Check sheet for the modelled part. Datum: model origin and axes. Units: mm. Give positions to 0.01 mm unless a question says otherwise; leave off trailing zeros. Write each loop counter-clockwise with the first axis right and the second up, starting at its lowest first coordinate (ties: lowest second). Pieces come first, ordered by that corner, then holes. Notation, with made-up numbers: M 76.5,64 L 117.5,64 A19 cw 117.5,101 Z; hole C -11.75,33.5 d5. An arc over 180 degrees is marked long. Use CSV: the item, a comma, the result in double quotes. Start each with the question number.
1. Scan lines: line 1 (X direction, y = 8.5, z = 0.75); line 2 (X direction, y = 17, z = 1.1); line 3 (X direction, y = -8.5, z = 0.3). Record each from-to range of solid material in increasing order.
2. Depth check by flat-ended pin: P1, Ø8, axis at x = 16.5, y = 24.5, coming from the +Z side. Enter the tip coordinate at first touch or a pass-through.
3. Cross-section at D-D, the plane x = -13. Enter the section's corners in (y, z), and give its area (3 significant figures).
4. Cross-section at A-A, the plane y = 0. Enter the section's corners in (x, z), and give its area (3 significant figures).
5. Cross-section at C-C, the plane y = -11. Enter the section's corners in (x, z).
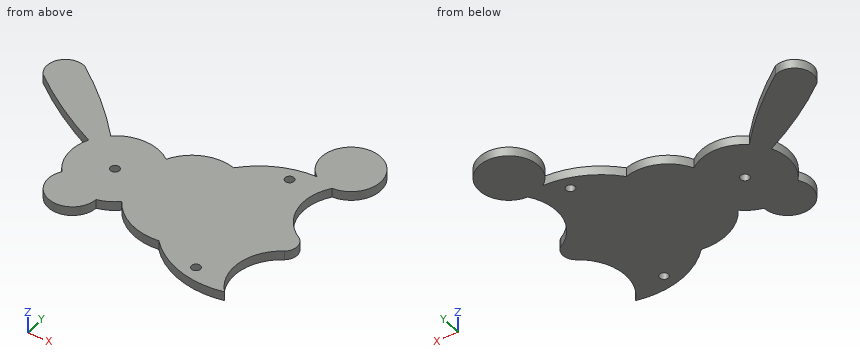
from build123d import *

# Parameters (mm, degrees)
F1_R     = 0.975
F1_R_2   = 5.495
F2_DEPTH = 2


# Not quite as in the source:
# - the program builds the solid bodies; features that only make, move or delete a surface that nothing else refers to are left out


with BuildPart() as f2:
    # F1 (on Top) → F2 (new body)
    with BuildSketch(Plane.XY):
        with BuildLine():
            ThreePointArc((8.3461548541, 12.451567302), (1.7252198574, 12.0948349613), (-3.0867358283, 7.5331334509))
            ThreePointArc((-3.0867358283, 7.5331334509), (-9.1504459177, 9.6196614304), (-15.1782928372, 7.431685066))
            ThreePointArc((-15.1782928372, 7.431685066), (-22.5381757879, 14.8578874844), (-30.6692253798, 21.4307401329))
            ThreePointArc((-30.6692253798, 21.4307401329), (-35.5250947404, 20.1584087851), (-35.4319922626, 15.1394819841))
            ThreePointArc((-35.4319922626, 15.1394819841), (-26.9109452732, 9.1280444677), (-17.7545223506, 4.1374991998))
            ThreePointArc((-17.7545223506, 4.1374991998), (-18.6125164693, -1.2164521529), (-16.4388114376, -6.1839420049))
            ThreePointArc((-16.4388114376, -6.1839420049), (-13.6846503599, -14.1883393203), (-6.7486233515, -9.3357823691))
            ThreePointArc((-6.7486233515, -9.3357823691), (-4.5490625181, -8.4916373097), (-2.6206436977, -7.1381789267))
            ThreePointArc((-2.6206436977, -7.1381789267), (2.5909813664, -11.6392406956), (9.3949967995, -12.7003565431))
            ThreePointArc((9.3949967995, -12.7003565431), (17.7901975829, -17.882711986), (27.6524089277, -18.1528814137))
            ThreePointArc((27.6524089277, -18.1528814137), (24.9662444476, -9.7026669711), (29.7177772104, -2.2163768254))
            ThreePointArc((29.7177772104, -2.2163768254), (30.8881367766, 0.1144698658), (29.7177772104, 2.4453165571))
            ThreePointArc((29.7177772104, 2.4453165571), (24.594325339, 9.3144076758), (26.3560396261, 17.700737901))
            ThreePointArc((26.3560396261, 17.700737901), (27.8220537541, 30.4194435664), (22.2002219007, 18.9168491704))
            ThreePointArc((22.2002219007, 18.9168491704), (14.5953140013, 17.1367848208), (8.3461548541, 12.451567302))
        make_face()
        with BuildLine():
            Line((-17.6755707347, -0.4939858073), (-12.0034380316, -0.4939858073))
            ThreePointArc((-12.0034380316, -0.4939858073), (-10.5336675739, -2.589890275), (-7.9799964747, -2.7682288675))
            Line((-7.9799964747, -2.7682288675), (-5.2005199999, -7.702828149))
            ThreePointArc((-5.2005199999, -7.702828149), (-5.9901385216, -8.0511163546), (-6.810625891, -8.3187029026))
            ThreePointArc((-6.810625891, -8.3187029026), (-7.2968984625, -8.4404428952), (-7.7895048721, -8.5332898913))
            ThreePointArc((-7.7895048721, -8.5332898913), (-13.3753397984, -13.2373782399), (-15.1250045058, -6.1473378715))
            ThreePointArc((-15.1250045058, -6.1473378715), (-15.4687321672, -5.7824640106), (-15.7903406401, -5.3979518136))
            ThreePointArc((-15.7903406401, -5.3979518136), (-17.1156764189, -3.0930980197), (-17.6755707347, -0.4939858073))
        make_face(mode=Mode.SUBTRACT)
        with Locations((-9.069736782, 0)):
            Circle(F1_R, mode=Mode.SUBTRACT)
        with Locations((19.3387361329, -15.2233078331)):
            Circle(F1_R, mode=Mode.SUBTRACT)
        with BuildLine():
            ThreePointArc((20.3872606575, 17.7804109262), (22.7170872685, 17.9218257414), (25.0456576674, 17.7610461256))
            ThreePointArc((25.0456576674, 17.7610461256), (25.1091906486, 17.7523846185), (25.172692422, 17.7434972003))
            ThreePointArc((25.172692422, 17.7434972003), (23.684740061, 8.8128379715), (29.166954709, 1.6075621931))
            ThreePointArc((29.166954709, 1.6075621931), (29.8880875558, 0.1007714549), (29.1453733807, -1.3954994316))
            ThreePointArc((29.1453733807, -1.3954994316), (24.1127403048, -8.7463736841), (25.8509191741, -17.4837349662))
            ThreePointArc((25.8509191741, -17.4837349662), (23.5178476173, -17.6742786032), (21.1797885868, -17.5602183711))
            ThreePointArc((21.1797885868, -17.5602183711), (20.0605128424, -12.3371922115), (16.6143622853, -16.4184698048))
            ThreePointArc((16.6143622853, -16.4184698048), (12.9131993659, -14.4284100321), (9.7748074556, -11.6338723113))
            ThreePointArc((9.7748074556, -11.6338723113), (2.6662624957, -10.5651214915), (-2.4218244994, -5.4872271944))
            ThreePointArc((-2.4218244994, -5.4872271944), (-3.341520275, -6.4414234179), (-4.3966137229, -7.2433639198))
            Line((-4.3966137229, -7.2433639198), (-7.1815796443, -2.2990188393))
            ThreePointArc((-7.1815796443, -2.2990188393), (-6.094920293, 0.0330432552), (-7.2331126554, 2.3403924495))
            Line((-7.2331126554, 2.3403924495), (-4.4863168152, 7.3004562466))
            ThreePointArc((-4.4863168152, 7.3004562466), (-3.5431905745, 6.6152616741), (-2.7011412367, 5.8090783073))
            ThreePointArc((-2.7011412367, 5.8090783073), (1.7884096787, 11.0249893996), (8.6656284498, 11.2812274136))
            ThreePointArc((8.6656284498, 11.2812274136), (11.9172089396, 14.3848906615), (15.8355289242, 16.5876774731))
            ThreePointArc((15.8355289242, 16.5876774731), (19.3270471679, 12.5448488398), (20.3872606575, 17.7804109262))
        make_face(mode=Mode.SUBTRACT)
        with BuildLine():
            ThreePointArc((-16.3638620166, 4.5934885503), (-26.0025688441, 9.741867589), (-34.9414590553, 16.0273045526))
            ThreePointArc((-34.9414590553, 16.0273045526), (-34.7398034138, 19.6908643856), (-31.1758954498, 20.5631577259))
            ThreePointArc((-31.1758954498, 20.5631577259), (-22.796689347, 13.7414479433), (-15.2552633126, 6.0036373591))
            ThreePointArc((-15.2552633126, 6.0036373591), (-10.598818784, 8.4832958354), (-5.3696469446, 7.7854823354))
            Line((-5.3696469446, 7.7854823354), (-8.119843394, 2.8192778422))
            ThreePointArc((-8.119843394, 2.8192778422), (-10.5540740424, 2.5782489983), (-11.9848002521, 0.5941632478))
            Line((-11.9848002521, 0.5941632478), (-17.6692350252, 0.5941632478))
            ThreePointArc((-17.6692350252, 0.5941632478), (-17.2642756667, 2.67468362), (-16.3638620166, 4.5934885503))
        make_face(mode=Mode.SUBTRACT)
        with Locations((18.5729401514, 15.4226861541)):
            Circle(F1_R, mode=Mode.SUBTRACT)
        with Locations((25.9979280814, 24.1858578784)):
            Circle(F1_R_2, mode=Mode.SUBTRACT)
        with BuildLine():
            ThreePointArc((25.172692422, 17.7434972003), (25.1091317315, 17.7519581241), (25.0456576674, 17.7610461256))
            ThreePointArc((25.0456576674, 17.7610461256), (22.7170872685, 17.9218257414), (20.3872606575, 17.7804109262))
            ThreePointArc((20.3872606575, 17.7804109262), (19.3270471679, 12.5448488398), (15.8355289242, 16.5876774731))
            ThreePointArc((15.8355289242, 16.5876774731), (11.9172089396, 14.3848906615), (8.6656284498, 11.2812274136))
            ThreePointArc((8.6656284498, 11.2812274136), (1.7884096787, 11.0249893996), (-2.7011412367, 5.8090783073))
            ThreePointArc((-2.7011412367, 5.8090783073), (-3.5431905745, 6.6152616741), (-4.4863168152, 7.3004562466))
            Line((-4.4863168152, 7.3004562466), (-7.2331126554, 2.3403924495))
            ThreePointArc((-7.2331126554, 2.3403924495), (-6.094920293, 0.0330432552), (-7.1815796443, -2.2990188393))
            Line((-7.1815796443, -2.2990188393), (-4.3966137229, -7.2433639198))
            ThreePointArc((-4.3966137229, -7.2433639198), (-3.341520275, -6.4414234179), (-2.4218244994, -5.4872271944))
            ThreePointArc((-2.4218244994, -5.4872271944), (2.6662624957, -10.5651214915), (9.7748074556, -11.6338723113))
            ThreePointArc((9.7748074556, -11.6338723113), (12.9131993659, -14.4284100321), (16.6143622853, -16.4184698048))
            ThreePointArc((16.6143622853, -16.4184698048), (20.0605128424, -12.3371922115), (21.1797885868, -17.5602183711))
            ThreePointArc((21.1797885868, -17.5602183711), (23.5178476173, -17.6742786032), (25.8509191741, -17.4837349662))
            ThreePointArc((25.8509191741, -17.4837349662), (24.1127403048, -8.7463736841), (29.1453733807, -1.3954994316))
            ThreePointArc((29.1453733807, -1.3954994316), (29.8880875558, 0.1007714549), (29.166954709, 1.6075621931))
            ThreePointArc((29.166954709, 1.6075621931), (23.684740061, 8.8128379715), (25.172692422, 17.7434972003))
        make_face()
        with BuildLine():
            ThreePointArc((-31.1758954498, 20.5631577259), (-34.7398034138, 19.6908643856), (-34.9414590553, 16.0273045526))
            ThreePointArc((-34.9414590553, 16.0273045526), (-26.0025688441, 9.741867589), (-16.3638620166, 4.5934885503))
            ThreePointArc((-16.3638620166, 4.5934885503), (-17.2642756667, 2.67468362), (-17.6692350252, 0.5941632478))
            Line((-17.6692350252, 0.5941632478), (-11.9848002521, 0.5941632478))
            ThreePointArc((-11.9848002521, 0.5941632478), (-10.5540740424, 2.5782489983), (-8.119843394, 2.8192778422))
            Line((-8.119843394, 2.8192778422), (-5.3696469446, 7.7854823354))
            ThreePointArc((-5.3696469446, 7.7854823354), (-10.598818784, 8.4832958354), (-15.2552633126, 6.0036373591))
            ThreePointArc((-15.2552633126, 6.0036373591), (-22.796689347, 13.7414479433), (-31.1758954498, 20.5631577259))
        make_face()
        with BuildLine():
            ThreePointArc((-7.9799964747, -2.7682288675), (-10.5336675739, -2.589890275), (-12.0034380316, -0.4939858073))
            Line((-12.0034380316, -0.4939858073), (-17.6755707347, -0.4939858073))
            ThreePointArc((-17.6755707347, -0.4939858073), (-17.1156764189, -3.0930980197), (-15.7903406401, -5.3979518136))
            ThreePointArc((-15.7903406401, -5.3979518136), (-15.4687321672, -5.7824640106), (-15.1250045058, -6.1473378715))
            ThreePointArc((-15.1250045058, -6.1473378715), (-13.3753397984, -13.2373782399), (-7.7895048721, -8.5332898913))
            ThreePointArc((-7.7895048721, -8.5332898913), (-7.2968984625, -8.4404428952), (-6.810625891, -8.3187029026))
            ThreePointArc((-6.810625891, -8.3187029026), (-5.9901385216, -8.0511163546), (-5.2005199999, -7.702828149))
            Line((-5.2005199999, -7.702828149), (-7.9799964747, -2.7682288675))
        make_face()
        with Locations((25.9979280814, 24.1858578784)):
            Circle(F1_R_2)
    extrude(amount=F2_DEPTH)


solid = f2.part
Worked answers:
1,line 1,"x = -25.89 to -16.14, -13.57 to -4.56, -2.54 to 24.81"
1,line 2,"x = -36.29 to -24.99, 14.31 to 25.89"
1,line 3,"x = -17.31 to -4.56, -1.59 to 25.19"
2,P1,"stops at z = 2"
3,outline,"M -14.36,0 L 8.78,0 L 8.78,2 L -14.36,2 Z"
3,area,"46.3 mm^2"
4,outline,"M -18.69,0 L -10.04,0 L -10.04,2 L -18.69,2 Z; M -8.09,0 L 30.89,0 L 30.89,2 L -8.09,2 Z"
4,area,"95.3 mm^2"
5,outline,"M -17.01,0 L -7.08,0 L -7.08,2 L -17.01,2 Z; M 1.39,0 L 24.88,0 L 24.88,2 L 1.39,2 Z"
